Could you check a few things on this model? Use its own coordinates, in mm. Face numbers are marked on the shaded views. A direction names the side the tool comes from. Round coordinates to 2 decimals unless told otherwise and drop trailing zeros. Put each result on its own line as item: value.
from build123d import *

# Parameters (mm, degrees)
BOSS_EXTRUDE1_DEPTH = 10


with BuildPart() as part:
    # Sketch1 → Boss-Extrude1 (new body)
    with BuildSketch(Plane.XY):
        with BuildLine():
            ThreePointArc((6.994301009, 16.632383564), (6.642138435, 16.776126687), (6.287024027, 16.912414331))
            ThreePointArc((6.287024027, 16.912414331), (5.167401268, 15.768670982), (4.351852136, 14.391505929))
            ThreePointArc((4.351852136, 14.391505929), (3.739075899, 14.562739143), (3.11960376, 14.707893537))
            ThreePointArc((3.11960376, 14.707893537), (3.068386931, 16.307606264), (2.63825659, 17.849258578))
            ThreePointArc((2.63825659, 17.849258578), (2.261410389, 17.900906476), (1.883559194, 17.944599031))
            ThreePointArc((1.883559194, 17.944599031), (1.083548848, 16.558349625), (0.636108713, 15.021631923))
            ThreePointArc((0.636108713, 15.021631923), (0, 15.035094277), (-0.636108713, 15.021631923))
            ThreePointArc((-0.636108713, 15.021631923), (-1.083548848, 16.558349625), (-1.883559194, 17.944599031))
            ThreePointArc((-1.883559194, 17.944599031), (-2.261410389, 17.900906476), (-2.63825659, 17.849258578))
            ThreePointArc((-2.63825659, 17.849258578), (-3.068386931, 16.307606264), (-3.11960376, 14.707893537))
            ThreePointArc((-3.11960376, 14.707893537), (-3.739075899, 14.562739143), (-4.351852136, 14.391505929))
            ThreePointArc((-4.351852136, 14.391505929), (-5.167401268, 15.768670982), (-6.287024027, 16.912414331))
            ThreePointArc((-6.287024027, 16.912414331), (-6.642138435, 16.776126687), (-6.994301009, 16.632383564))
            ThreePointArc((-6.994301009, 16.632383564), (-7.027524675, 15.032196025), (-6.679300055, 13.470004109))
            ThreePointArc((-6.679300055, 13.470004109), (-7.243211909, 13.17535355), (-7.794152684, 12.85710869))
            ThreePointArc((-7.794152684, 12.85710869), (-8.926566862, 13.988188748), (-10.295452017, 14.817560439))
            ThreePointArc((-10.295452017, 14.817560439), (-10.605516495, 14.597241161), (-10.910867773, 14.37043472))
            ThreePointArc((-10.910867773, 14.37043472), (-10.545097198, 12.812257626), (-9.819311364, 11.385744783))
            ThreePointArc((-9.819311364, 11.385744783), (-10.292230275, 10.960112038), (-10.746717955, 10.514852026))
            ThreePointArc((-10.746717955, 10.514852026), (-12.124843431, 11.32877717), (-13.656978894, 11.79166473))
            ThreePointArc((-13.656978894, 11.79166473), (-13.902510949, 11.501157287), (-14.141864588, 11.205538613))
            ThreePointArc((-14.141864588, 11.205538613), (-13.400082482, 9.787277961), (-12.342339226, 8.586077239))
            ThreePointArc((-12.342339226, 8.586077239), (-12.694549961, 8.056206379), (-13.024027412, 7.511908539))
            ThreePointArc((-13.024027412, 7.511908539), (-14.561271495, 7.957536859), (-16.16038756, 8.024855359))
            ThreePointArc((-16.16038756, 8.024855359), (-16.32595951, 7.682413402), (-16.48427604, 7.336557303))
            ThreePointArc((-16.48427604, 7.336557303), (-15.413091302, 6.147327625), (-14.089852523, 5.246914884))
            ThreePointArc((-14.089852523, 5.246914884), (-14.299224386, 4.646099644), (-14.482989328, 4.036964211))
            ThreePointArc((-14.482989328, 4.036964211), (-16.082761318, 4.08629524), (-17.648379642, 3.753814812))
            ThreePointArc((-17.648379642, 3.753814812), (-17.723587993, 3.38095523), (-17.790919803, 3.006593116))
            ThreePointArc((-17.790919803, 3.006593116), (-16.457638909, 2.121118087), (-14.952048567, 1.57806957))
            ThreePointArc((-14.952048567, 1.57806957), (-15.005425953, 0.944061381), (-15.03193176, 0.308362575))
            ThreePointArc((-15.03193176, 0.308362575), (-16.593712099, -0.041703336), (-18.027459124, -0.753091724))
            ThreePointArc((-18.027459124, -0.753091724), (-18.00757826, -1.132940794), (-17.979694645, -1.512286374))
            ThreePointArc((-17.979694645, -1.512286374), (-16.468092537, -2.038369101), (-14.87475241, -2.189931658))
            ThreePointArc((-14.87475241, -2.189931658), (-14.768781422, -2.817295731), (-14.636362636, -3.439614616))
            ThreePointArc((-14.636362636, -3.439614616), (-16.062018922, -4.167081539), (-17.27380705, -5.212678738))
            ThreePointArc((-17.27380705, -5.212678738), (-17.160086157, -5.575649981), (-17.038739148, -5.936143349))
            ThreePointArc((-17.038739148, -5.936143349), (-15.443795346, -6.069778062), (-13.862820853, -5.820331426))
            ThreePointArc((-13.862820853, -5.820331426), (-13.604160038, -6.40163179), (-13.321137019, -6.97146817))
            ThreePointArc((-13.321137019, -6.97146817), (-14.521090024, -8.030626683), (-15.43477815, -9.344733977))
            ThreePointArc((-15.43477815, -9.344733977), (-15.23436273, -9.668020574), (-15.027177006, -9.987010606))
            ThreePointArc((-15.027177006, -9.987010606), (-13.449107694, -9.719800545), (-11.979837279, -9.085018366))
            ThreePointArc((-11.979837279, -9.085018366), (-11.584739247, -9.58372978), (-11.168895371, -10.06527874))
            ThreePointArc((-11.168895371, -10.06527874), (-12.067747635, -11.389578018), (-12.625925373, -12.889625211))
            ThreePointArc((-12.625925373, -12.889625211), (-12.351408265, -13.152913878), (-12.071402067, -13.410357257))
            ThreePointArc((-12.071402067, -13.410357257), (-10.609363144, -12.759092212), (-9.344116469, -11.778860189))
            ThreePointArc((-9.344116469, -11.778860189), (-8.837406683, -12.163646782), (-8.314870951, -12.526650829))
            ThreePointArc((-8.314870951, -12.526650829), (-8.85614428, -14.032880278), (-9.023739271, -15.624613889))
            ThreePointArc((-9.023739271, -15.624613889), (-8.692369394, -15.81136123), (-8.35713654, -15.991081842))
            ThreePointArc((-8.35713654, -15.991081842), (-7.102993289, -14.996683191), (-6.121270456, -13.732592906))
            ThreePointArc((-6.121270456, -13.732592906), (-5.534787355, -13.979277122), (-4.938392608, -14.200927377))
            ThreePointArc((-4.938392608, -14.200927377), (-5.088076809, -15.794445061), (-4.854558443, -17.377850613))
            ThreePointArc((-4.854558443, -17.377850613), (-4.487156985, -17.476322606), (-4.117761389, -17.567027943))
            ThreePointArc((-4.117761389, -17.567027943), (-3.150316243, -16.291977412), (-2.513802508, -14.823456307))
            ThreePointArc((-2.513802508, -14.823456307), (-1.884396983, -14.916538068), (-1.251616896, -14.982907431))
            ThreePointArc((-1.251616896, -14.982907431), (-1.000306759, -16.563586773), (-0.380347854, -18.039173072))
            ThreePointArc((-0.380347854, -18.039173072), (0, -18.043182358), (0.380347854, -18.039173072))
            ThreePointArc((0.380347854, -18.039173072), (1.000306759, -16.563586773), (1.251616896, -14.982907431))
            ThreePointArc((1.251616896, -14.982907431), (1.884396983, -14.916538068), (2.513802508, -14.823456307))
            ThreePointArc((2.513802508, -14.823456307), (3.150316243, -16.291977412), (4.117761389, -17.567027943))
            ThreePointArc((4.117761389, -17.567027943), (4.487156985, -17.476322606), (4.854558443, -17.377850613))
            ThreePointArc((4.854558443, -17.377850613), (5.088076809, -15.794445061), (4.938392608, -14.200927377))
            ThreePointArc((4.938392608, -14.200927377), (5.534787355, -13.979277122), (6.121270456, -13.732592906))
            ThreePointArc((6.121270456, -13.732592906), (7.102993289, -14.996683191), (8.35713654, -15.991081842))
            ThreePointArc((8.35713654, -15.991081842), (8.692369394, -15.81136123), (9.023739271, -15.624613889))
            ThreePointArc((9.023739271, -15.624613889), (8.85614428, -14.032880278), (8.314870951, -12.526650829))
            ThreePointArc((8.314870951, -12.526650829), (8.837406683, -12.163646782), (9.344116469, -11.778860189))
            ThreePointArc((9.344116469, -11.778860189), (10.609363144, -12.759092212), (12.071402067, -13.410357257))
            ThreePointArc((12.071402067, -13.410357257), (12.351408265, -13.152913878), (12.625925373, -12.889625211))
            ThreePointArc((12.625925373, -12.889625211), (12.067747635, -11.389578018), (11.168895371, -10.06527874))
            ThreePointArc((11.168895371, -10.06527874), (11.584739247, -9.58372978), (11.979837279, -9.085018366))
            ThreePointArc((11.979837279, -9.085018366), (13.449107694, -9.719800545), (15.027177006, -9.987010606))
            ThreePointArc((15.027177006, -9.987010606), (15.23436273, -9.668020574), (15.43477815, -9.344733977))
            ThreePointArc((15.43477815, -9.344733977), (14.521090024, -8.030626683), (13.321137019, -6.97146817))
            ThreePointArc((13.321137019, -6.97146817), (13.604160038, -6.40163179), (13.862820853, -5.820331426))
            ThreePointArc((13.862820853, -5.820331426), (15.443795346, -6.069778062), (17.038739148, -5.936143349))
            ThreePointArc((17.038739148, -5.936143349), (17.160086157, -5.575649981), (17.27380705, -5.212678738))
            ThreePointArc((17.27380705, -5.212678738), (16.062018922, -4.167081539), (14.636362636, -3.439614616))
            ThreePointArc((14.636362636, -3.439614616), (14.768781422, -2.817295731), (14.87475241, -2.189931658))
            ThreePointArc((14.87475241, -2.189931658), (16.468092537, -2.038369101), (17.979694645, -1.512286374))
            ThreePointArc((17.979694645, -1.512286374), (18.00757826, -1.132940794), (18.027459124, -0.753091724))
            ThreePointArc((18.027459124, -0.753091724), (16.593712099, -0.041703336), (15.03193176, 0.308362575))
            ThreePointArc((15.03193176, 0.308362575), (15.005425953, 0.944061381), (14.952048567, 1.57806957))
            ThreePointArc((14.952048567, 1.57806957), (16.457638909, 2.121118087), (17.790919803, 3.006593116))
            ThreePointArc((17.790919803, 3.006593116), (17.723587993, 3.38095523), (17.648379642, 3.753814812))
            ThreePointArc((17.648379642, 3.753814812), (16.082761318, 4.08629524), (14.482989328, 4.036964211))
            ThreePointArc((14.482989328, 4.036964211), (14.299224386, 4.646099644), (14.089852523, 5.246914884))
            ThreePointArc((14.089852523, 5.246914884), (15.413091302, 6.147327625), (16.48427604, 7.336557303))
            ThreePointArc((16.48427604, 7.336557303), (16.32595951, 7.682413402), (16.16038756, 8.024855359))
            ThreePointArc((16.16038756, 8.024855359), (14.561271495, 7.957536859), (13.024027412, 7.511908539))
            ThreePointArc((13.024027412, 7.511908539), (12.694549961, 8.056206379), (12.342339226, 8.586077239))
            ThreePointArc((12.342339226, 8.586077239), (13.400082482, 9.787277961), (14.141864588, 11.205538613))
            ThreePointArc((14.141864588, 11.205538613), (13.902510949, 11.501157287), (13.656978894, 11.79166473))
            ThreePointArc((13.656978894, 11.79166473), (12.124843431, 11.32877717), (10.746717955, 10.514852026))
            ThreePointArc((10.746717955, 10.514852026), (10.292230275, 10.960112038), (9.819311364, 11.385744783))
            ThreePointArc((9.819311364, 11.385744783), (10.545097198, 12.812257626), (10.910867773, 14.37043472))
            ThreePointArc((10.910867773, 14.37043472), (10.605516495, 14.597241161), (10.295452017, 14.817560439))
            ThreePointArc((10.295452017, 14.817560439), (8.926566862, 13.988188748), (7.794152684, 12.85710869))
            ThreePointArc((7.794152684, 12.85710869), (7.243211909, 13.17535355), (6.679300055, 13.470004109))
            ThreePointArc((6.679300055, 13.470004109), (7.027524675, 15.032196025), (6.994301009, 16.632383564))
        make_face()
        with BuildLine():
            Line((-1.542724862, 1.35), (1.542724862, 1.35))
            ThreePointArc((1.542724862, 1.35), (0, -2.05), (-1.542724862, 1.35))
        make_face(mode=Mode.SUBTRACT)
    extrude(amount=BOSS_EXTRUDE1_DEPTH)


solid = part.part
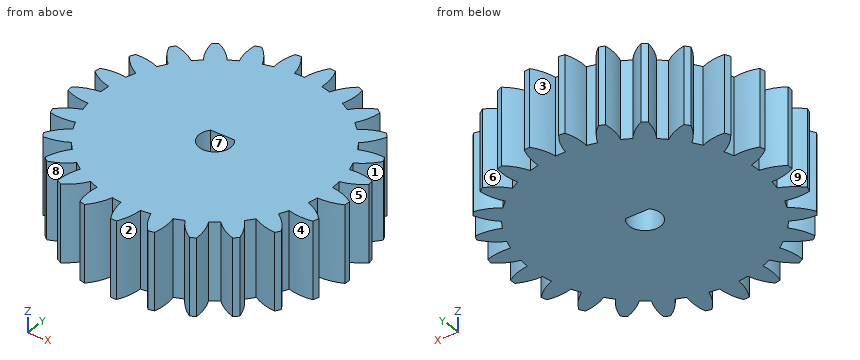
(1) Please list where these lines run through material, in increasing order: probe 1 along Y at (x, z) = (0, 5.75); probe 2 along X at (y, z) = (-12, 2.25); probe 3 along X at (y, z) = (1, 7). Write a range as from..to.
Values found:
probe 1: y = -18.04..-2.05, 1.35..15.04
probe 2: x = -12.34..-9.58, -9.06..9.06, 9.58..12.34
probe 3: x = -15..-1.79, 1.79..15
(2) If we mould it in two halves opening along Y, with no side actions, what happens to the marked faces 1, 2, 3 and 4? For each: pulls with the +Y half, pulls with the -Y half, needs draft (parallel to the pull), parting line crosses it, or undercut.
Values found:
face 1: undercut
face 2: pulls with the -Y half
face 3: pulls with the +Y half
face 4: undercut
(3) I'm going to push flat-ended pins straight in: pin 1 (6 mm diameter, centred on x = -9, z = 2, fed in from +Y); pin 2 (4 mm diameter, centred on y = -11, z = 8, fed in from -X); pin 3 (6 mm diameter, centred on y = -7.5, z = 6.5, fed in from +X). Where does each tip first touch, or does it pass through?
Values found:
pin 1: stops at y = 16.91
pin 2: stops at x = -15.43
pin 3: stops at x = 17.27
(4) For the marked faces 5, 6, 7, 8 and 9, which set-ups out of +Z, -Z, +X, -X, +Y, -Y let a thin tool reach every point of the face, with its end or its side?
Values found:
face 5: +Z, -Z, +X
face 6: +Z, -Z, +Y
face 7: +Z, -Z
face 8: +Z, -Z, -Y
face 9: +Z, -Z, -X
